```python
from build123d import *

# Parameters (mm, degrees)
BOSS_EXTRUDE1_DEPTH = 90
CUT_EXTRUDE1_DEPTH  = 90
SKETCH3_W           = 36
SKETCH3_H           = 75.56624327
BOSS_EXTRUDE2_DEPTH = 10
SKETCH4_W           = 24
SKETCH4_H           = 75.56624327
BOSS_EXTRUDE3_DEPTH = 35
SKETCH5_W           = 24
SKETCH5_H           = 32
CUT_EXTRUDE2_DEPTH  = 20
CUT_EXTRUDE3_DEPTH  = 440
SKETCH9_R           = 10
CUT_EXTRUDE6_DEPTH  = 440
SKETCH11_R          = 6
CUT_EXTRUDE7_DEPTH  = 440
CUT_EXTRUDE8_DEPTH  = 440
CUT_EXTRUDE9_DEPTH  = 440
CUT_EXTRUDE10_DEPTH = 89
CUT_EXTRUDE10_TAPER = 1
BOSS_EXTRUDE4_DEPTH = 24


with BuildPart() as part:
    # Sketch1 → Boss-Extrude1 (new body)
    with BuildSketch(Plane.XY):
        with BuildLine():
            Line((-30, 12.5), (30, 12.5))
            ThreePointArc((30, 12.5), (42.5, 0), (30, -12.5))
            Line((30, -12.5), (-30, -12.5))
            ThreePointArc((-30, -12.5), (-42.5, 0), (-30, 12.5))
        make_face()
    extrude(amount=BOSS_EXTRUDE1_DEPTH)

    # Sketch2 → Cut-Extrude1 (cut)
    with BuildSketch(Plane(origin=(42.5, 0, 0), x_dir=(0, 0, -1), z_dir=(1, 0, 0))):
        Polygon((0, -12.5), (-14.43375673, 12.5), (0, 12.5), align=None)
    extrude(amount=-CUT_EXTRUDE1_DEPTH, mode=Mode.SUBTRACT)

    # Sketch3 → Boss-Extrude2 (add)
    with BuildSketch(Plane(origin=(0, 12.5, 0), x_dir=(1, 0, 0), z_dir=(0, 1, 0))):
        with Locations((0, -52.216878365)):
            Rectangle(SKETCH3_W, SKETCH3_H)
    extrude(amount=BOSS_EXTRUDE2_DEPTH)

    # Sketch4 → Boss-Extrude3 (add)
    with BuildSketch(Plane(origin=(0, 22.5, 0), x_dir=(1, 0, 0), z_dir=(0, 1, 0))):
        with Locations((0, -52.216878365)):
            Rectangle(SKETCH4_W, SKETCH4_H)
    extrude(amount=BOSS_EXTRUDE3_DEPTH)

    # Sketch5 → Cut-Extrude2 (cut)
    with BuildSketch(Plane(origin=(0, 57.5, 0), x_dir=(1, 0, 0), z_dir=(0, 1, 0))):
        with Locations((0, -74)):
            Rectangle(SKETCH5_W, SKETCH5_H)
    extrude(amount=-CUT_EXTRUDE2_DEPTH, mode=Mode.SUBTRACT)

    # Sketch6 → Cut-Extrude3 (cut)
    with BuildSketch(Plane(origin=(42.5, 0, 0), x_dir=(0, 0, -1), z_dir=(1, 0, 0))):
        Polygon((-14.43375673, 12.5), (-40.414518843, 57.5), (-14.43375673, 57.5), align=None)
    extrude(amount=-CUT_EXTRUDE3_DEPTH, mode=Mode.SUBTRACT)

    # Sketch9 → Cut-Extrude6 (cut)
    with BuildSketch(Plane.XY.offset(90)):
        with Locations((0, 12.5)):
            Circle(SKETCH9_R)
    extrude(amount=-CUT_EXTRUDE6_DEPTH, mode=Mode.SUBTRACT)

    # Sketch11 → Cut-Extrude7 (cut)
    with BuildSketch(Plane(origin=(0, 37.5, 0), x_dir=(1, 0, 0), z_dir=(0, 1, 0))):
        with Locations((0, -78)):
            Circle(SKETCH11_R)
    extrude(amount=-CUT_EXTRUDE7_DEPTH, mode=Mode.SUBTRACT)

    # Sketch12 → Cut-Extrude8 (cut)
    with BuildSketch(Plane.ZY.offset(12)):
        with BuildLine():
            Line((55, 57.5), (58, 57.5))
            Line((58, 57.5), (58, 54.5))
            ThreePointArc((58, 54.5), (57.121320344, 56.621320344), (55, 57.5))
        make_face()
    extrude(amount=-CUT_EXTRUDE8_DEPTH, mode=Mode.SUBTRACT)

    # Sketch13 → Cut-Extrude9 (cut)
    with BuildSketch(Plane.ZY.offset(12)):
        with BuildLine():
            Line((87, 37.5), (90, 37.5))
            Line((90, 37.5), (90, 34.5))
            ThreePointArc((90, 34.5), (89.121320344, 36.621320344), (87, 37.5))
        make_face()
    extrude(amount=-CUT_EXTRUDE9_DEPTH, mode=Mode.SUBTRACT)

    # Sketch14 → Cut-Extrude10 (cut)
    with BuildSketch(Plane(origin=(0, -3.125, 5.412658774), x_dir=(-1, 0, 0), z_dir=(0, 0.5, -0.866025404))):
        Polygon((-6, 34.174682453), (6, 34.174682453), (0, 49.174682453), align=None)
    extrude(amount=-CUT_EXTRUDE10_DEPTH, taper=CUT_EXTRUDE10_TAPER, mode=Mode.SUBTRACT)

    # Sketch16 → Boss-Extrude4 (add)
    with BuildSketch(Plane(origin=(12, 0, 0), x_dir=(0, 0, -1), z_dir=(1, 0, 0))):
        with BuildLine():
            Line((-61, 37.5), (-58, 37.5))
            Line((-58, 37.5), (-58, 40.5))
            ThreePointArc((-58, 40.5), (-58.878679656, 38.378679656), (-61, 37.5))
        make_face()
    extrude(amount=-BOSS_EXTRUDE4_DEPTH)


solid = part.part
```
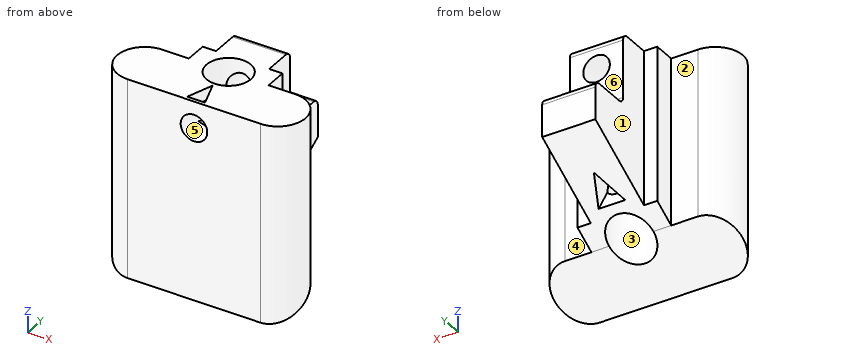
Check sheet for the modelled part. Datum: model origin and axes. Units: mm. Face numbers are marked on the shaded views. A direction names the side the tool comes from. Give positions to 0.01 mm unless a question says otherwise; leave off trailing zeros. Loops run counter-clockwise (first coordinate to the right, second up) from the corner with the lowest first, then second, coordinate; pieces in that order, holes last. Notation, with made-up numbers: M -14.5,8 L -4.5,8 A24 cw -4.5,21 Z; hole C -5.5,10 d1. An arc over 180 degrees is marked long. Answer as CSV lines item,"result".
Item 1: Draft check along X on the marked faces 1, 2 and 3. Enter one of: pulls with the +X half, pulls with the -X half, needs draft (parallel to the pull), parting line crosses it, or undercut.
Reply:
face 1,"pulls with the -X half"
face 2,"needs draft"
face 3,"undercut"
Item 2: Sectioned sample at A-A, the plane z = 78. Enter the section's corners in (x, y).
Reply:
outline,"M -30,-12.5 L -6,-12.5 L -6,4.5 A10 cw -6,20.5 L -6,37.5 L -12,37.5 L -12,22.5 L -18,22.5 L -18,12.5 L -30,12.5 A12.5 ccw Z; M 6,-12.5 L 30,-12.5 A12.5 ccw 30,12.5 L 18,12.5 L 18,22.5 L 12,22.5 L 12,37.5 L 6,37.5 L 6,20.5 A10 cw 6,4.5 Z"
Item 3: Sectioned sample at B-B, the plane y = 10.5. Enter the section's corners in (x, z).
Reply:
outline,"M -36.78,13.28 L -9.8,13.28 L -9.8,90 L -36.78,90 Z; M 9.8,13.28 L 36.78,13.28 L 36.78,90 L 9.8,90 Z"
Item 4: Sectioned sample at C-C, the plane x = -21.5. Enter the section's corners in (y, z).
Reply:
outline,"M -12.5,0 L 12.5,14.43 L 12.5,90 L -12.5,90 Z"
Item 5: Sectioned sample at D-D, the plane y = 42.5. Enter the section's corners in (x, z).
Reply:
outline,"M -12,31.75 L 12,31.75 L 12,58 L -12,58 Z"
Item 6: Scan lines: L1, parallel to X at y = 26, z = 78; L2, parallel to X at y = 11, z = 42; L3, parallel to Y at x = 8, z = 78.5. Record each from-to range of solid material in increasing order.
Reply:
L1,"-12 to -6, 6 to 12"
L2,"-35.94 to -9.89, 9.89 to 35.94"
L3,"-12.5 to 6.5, 18.5 to 37.5"
Item 7: Depth check by flat-ended pin: pin 1 Ø3 at (y, z) = (19.5, 37.5) entering from +X; pin 2 Ø3.5 at (x, z) = (-24, 37.5) entering from +Y; pin 3 Ø4 at (y, z) = (41.5, 27) entering from +X; pin 4 Ø12 at (y, z) = (34.5, 32.5) entering from -X. Enter the tip coordinate at first touch or a pass-through.
Reply:
pin 1,"x = 18"
pin 2,"y = 12.5"
pin 3,"through"
pin 4,"x = -12"
Item 8: Set-up check for the marked faces 4, 5 and 6: record each of +Z, -Z, +X, -X, +Y, -Y from which the full face is reachable in a straight line by a thin tool's end or side.
Reply:
face 4,"+Z, -Z, +X, +Y"
face 5,"+Y, -Y"
face 6,"+Z, +X, -X, +Y"
